Source: CAD feature listing. Evaluate the final solid. Frame: model axes, mm. Round coordinates to 2 decimals unless told otherwise and drop trailing zeros. Loops run counter-clockwise (first coordinate to the right, second up) from the corner with the lowest first, then second, coordinate; pieces in that order, holes last.
(1) Section D-D, the plane z = -207. Return the cut outline in (x, y).
(2) Section B-B, the plane z = -47. Return the cut outline in (x, y), plus the area to 3 significant figures.
(3) First-contact query: pin 1 Ø2.5 at (y, z) = (3, -191) entering from +X; pin 2 Ø2 at (x, y) = (28.5, 3) entering from -Z; pin 3 Ø1.4 at (y, z) = (1.5, -241.5) entering from -X. Flat tips, straight axial feed; report the tip coordinate or a pass-through.
(4) Section C-C, the plane x = 186. Return the cut outline in (y, z), plus the area to 3 significant figures.
(5) Section A-A, the plane x = 238. Return the cut outline in (y, z), plus the area to 3 significant figures.
(6) Material intervals for probe 1 along Z at (x, y) = (169, 1.35); probe 2 along Z at (x, y) = (97.5, 1.2); probe 3 along X at (y, z) = (3.6, -237.5), sorted ascending.
```python
from build123d import *

# Parameters (mm, degrees)
SKETCH1_W            = 254
SKETCH1_H            = 254
BOSS_EXTRUDE1_DEPTH  = 4.800000052
CUT_EXTRUDE2_DEPTH   = 360.242313767
CUT_EXTRUDE3_DEPTH   = 4.826
CUT_EXTRUDE5_DEPTH   = 4.826
CUT_EXTRUDE6_DEPTH   = 4.826
SKETCH16_OUTSIDE_W   = 327.848
SKETCH16_OUTSIDE_H   = 327.848
CUT_EXTRUDE8_DEPTH   = 360.242313767
SKETCH17_OUTSIDE_W   = 327.848
SKETCH17_OUTSIDE_H   = 327.848
CUT_EXTRUDE17_DEPTH  = 360.242313767
SKETCH18_OUTSIDE_W   = 327.848
SKETCH18_OUTSIDE_H   = 327.848
CUT_EXTRUDE18_DEPTH  = 216.155906991
SKETCH19_OUTSIDE_W   = 327.734
SKETCH19_OUTSIDE_H   = 327.834
SKETCH19_OUTSIDE_W_2 = 4.500000144
SKETCH19_OUTSIDE_H_2 = 16.933333333
CUT_EXTRUDE19_DEPTH  = 364.309275828
SKETCH32_W           = 4.800000052
SKETCH32_H           = 76.2
CUT_EXTRUDE22_DEPTH  = 25.4
CUT_EXTRUDE23_DEPTH  = 216.155906991
SKETCH34_W           = 4.800000052
SKETCH34_H           = 76.2
CUT_EXTRUDE24_DEPTH  = 25.4
SKETCH36_W           = 4.500000144
SKETCH36_H           = 16.933333333
CUT_EXTRUDE26_DEPTH  = 364.309275828
SKETCH37_W           = 4.500000144
SKETCH37_H           = 25.4
CUT_EXTRUDE27_DEPTH  = 360.171616324
SKETCH48_W           = 4.500000144
SKETCH48_H           = 25.4
CUT_EXTRUDE34_DEPTH  = 360.171616324
SKETCH50_R           = 1.4
CUT_EXTRUDE35_DEPTH  = 506.24041807
SKETCH51_R           = 1.1
CUT_EXTRUDE36_DEPTH  = 1021.904407936


with BuildPart() as part:
    # Sketch1 → Boss-Extrude1 (new body)
    with BuildSketch(Plane(origin=(0, 0, 0), x_dir=(1, 0, 0), z_dir=(0, 1, 0))):
        with Locations((127, 127)):
            Rectangle(SKETCH1_W, SKETCH1_H)
    extrude(amount=BOSS_EXTRUDE1_DEPTH)

    # Sketch4 → Cut-Extrude2 (cut, through all)
    with BuildSketch(Plane(origin=(0, 4.800000052, 0), x_dir=(1, 0, 0), z_dir=(0, 1, 0))):
        Polygon((76.2, 254), (0, 177.8), (0, 254), align=None)
    extrude(amount=-CUT_EXTRUDE2_DEPTH, mode=Mode.SUBTRACT)

    # Sketch5 → Cut-Extrude3 (cut)
    with BuildSketch(Plane(origin=(0, 4.800000052, 0), x_dir=(1, 0, 0), z_dir=(0, 1, 0))):
        Polygon((177.8, 254), (254, 177.8), (254, 254), align=None)
    extrude(amount=-CUT_EXTRUDE3_DEPTH, mode=Mode.SUBTRACT)

    # Sketch9 → Cut-Extrude5 (cut)
    with BuildSketch(Plane(origin=(0, 4.800000052, 0), x_dir=(1, 0, 0), z_dir=(0, 1, 0))):
        Polygon((0, 76.2), (0, 0), (76.2, 0), align=None)
    extrude(amount=-CUT_EXTRUDE5_DEPTH, mode=Mode.SUBTRACT)

    # Sketch11 → Cut-Extrude6 (cut)
    with BuildSketch(Plane(origin=(0, 4.800000052, 0), x_dir=(1, 0, 0), z_dir=(0, 1, 0))):
        Polygon((254, 76.2), (254, 0), (177.8, 0), align=None)
    extrude(amount=-CUT_EXTRUDE6_DEPTH, mode=Mode.SUBTRACT)

    # Sketch16 outside → Cut-Extrude8 (cut, through all)
    # profile 1 of 2: a face of its own
    with BuildSketch(Plane.XZ):
        with Locations((127, -127)):
            Rectangle(SKETCH16_OUTSIDE_W, SKETCH16_OUTSIDE_H)
        Polygon((254, -76.2), (177.8, 0), (76.2, 0), (0, -76.2), (0, -177.8), (76.2, -254), (177.8, -254), (254, -177.8), align=None, mode=Mode.SUBTRACT)
    # profile 2 of 2: a face of its own
    with BuildSketch(Plane.XZ):
        Polygon((154.05, -237.45), (152.4, -239.09956871), (152.4, -247.65), (157.899988492, -247.65), (157.899988492, -247.233680101), (157.899988492, -246.283680101), (157.899988492, -243.349999982), (157.899988492, -243.025), (157.899988492, -242.075), (157.899988492, -241.750000018), (157.899988492, -240.049999963), (157.899991793, -239.09957201), (156.249995092, -237.45), align=None)
    extrude(amount=-CUT_EXTRUDE8_DEPTH, mode=Mode.SUBTRACT)

    # Sketch17 outside → Cut-Extrude17 (cut, through all)
    # profile 1 of 2: a face of its own
    with BuildSketch(Plane.XZ):
        with Locations((127, -127)):
            Rectangle(SKETCH17_OUTSIDE_W, SKETCH17_OUTSIDE_H)
        Polygon((254, -76.2), (177.8, 0), (76.2, 0), (0, -76.2), (0, -177.8), (76.2, -254), (177.8, -254), (254, -177.8), align=None, mode=Mode.SUBTRACT)
    # profile 2 of 2: a face of its own
    with BuildSketch(Plane.XZ):
        Polygon((125.900002454, -218.4), (128.099997546, -218.4), (129.749994246, -220.04956871), (129.749994246, -220.999999963), (129.749994246, -222.700000018), (129.749994246, -223.025), (129.749994246, -223.975), (129.749994246, -224.299999982), (129.749994246, -227.233680101), (129.749994246, -228.183680101), (129.749994246, -228.6), (124.250005754, -228.6), (124.250005754, -228.183680101), (124.250005754, -228.15), (124.250005754, -227.233680101), (124.250005754, -224.299999982), (124.250005754, -223.975), (124.250005754, -223.025), (124.250005754, -222.700000018), (124.250005754, -220.999999963), (124.250005754, -220.04956871), align=None)
    extrude(amount=-CUT_EXTRUDE17_DEPTH, mode=Mode.SUBTRACT)

    # Sketch18 outside → Cut-Extrude18 (cut, through all)
    # profile 1 of 2: a face of its own
    with BuildSketch(Plane(origin=(166.661666982, 4.800000052, -135.988650526), x_dir=(1, 0, 0), z_dir=(0, 1, 0))):
        with Locations((-39.662, -8.989)):
            Rectangle(SKETCH18_OUTSIDE_W, SKETCH18_OUTSIDE_H)
        Polygon((-90.561667036, -135.988650526), (11.038332964, -135.988650526), (87.238332964, -59.788650526), (87.238332964, 41.811349474), (11.038332964, 118.011349474), (-90.561667036, 118.011349474), (-166.761667036, 41.811349474), (-166.761667036, -59.788650526), align=None, mode=Mode.SUBTRACT)
    # profile 2 of 2: a face of its own
    with BuildSketch(Plane(origin=(166.661666982, 4.800000052, -135.988650526), x_dir=(1, 0, 0), z_dir=(0, 1, 0))):
        Polygon((-65.461678544, 103.110918185), (-65.461678544, 111.661349474), (-70.961667036, 111.661349474), (-70.812431754, 103.061695826), (-69.211666982, 101.461349474), (-67.01167189, 101.461349474), align=None)
    extrude(amount=-CUT_EXTRUDE18_DEPTH, mode=Mode.SUBTRACT)

    # Sketch19 outside → Cut-Extrude19 (cut, through all)
    # profile 1 of 3: a face of its own
    with BuildSketch(Plane(origin=(277.632305151, 0, -234.288055689), x_dir=(1, 0, 0), z_dir=(0, -1, 0))):
        with Locations((-150.682, 107.288)):
            Rectangle(SKETCH19_OUTSIDE_W, SKETCH19_OUTSIDE_H)
        Polygon((-23.632305151, 158.088055689), (-99.832305151, 234.288055689), (-201.432305151, 234.288055689), (-277.632305151, 158.088055689), (-277.632305151, 56.488055689), (-201.432305151, -19.711944311), (-99.832305151, -19.711944311), (-23.632305151, 56.488055689), align=None, mode=Mode.SUBTRACT)
    # profile 2 of 3: a face of its own
    with BuildSketch(Plane(origin=(277.632305151, 0, -234.288055689), x_dir=(1, 0, 0), z_dir=(0, -1, 0))):
        with Locations((-54.584305223, 132.68805569)):
            Rectangle(SKETCH19_OUTSIDE_W_2, SKETCH19_OUTSIDE_H_2)
    # profile 3 of 3: a face of its own
    with BuildSketch(Plane(origin=(277.632305151, 0, -234.288055689), x_dir=(1, 0, 0), z_dir=(0, -1, 0))):
        with Locations((-54.584305223, 98.821389023)):
            Rectangle(SKETCH19_OUTSIDE_W_2, SKETCH19_OUTSIDE_H_2)
    cut_extrude19 = extrude(amount=-CUT_EXTRUDE19_DEPTH, mode=Mode.SUBTRACT)

    # Mirror2: Cut-Extrude19 across plane
    add(cut_extrude19.mirror(Plane(origin=(126.949999973, 0, 0), x_dir=(0, 0, 1), z_dir=(1, 0, 0))), mode=Mode.SUBTRACT)

    # Sketch32 → Cut-Extrude22 (cut)
    with BuildSketch(Plane(origin=(254, 6.738807757, -234.288055689), x_dir=(0, 1, 0), z_dir=(1, 0, 0))):
        with Locations((-4.338807731, 107.288055689)):
            Rectangle(SKETCH32_W, SKETCH32_H)
    extrude(amount=-CUT_EXTRUDE22_DEPTH, mode=Mode.SUBTRACT)

    # Sketch33 → Cut-Extrude23 (cut, through all)
    with BuildSketch(Plane(origin=(166.661666982, 0, -135.988650526), x_dir=(1, 0, 0), z_dir=(0, -1, 0))):
        Polygon((-42.582666982, 122.75320968), (-42.582666982, 125.686889799), (-42.582666982, 126.011889781), (-42.582666982, 126.961889781), (-42.582666982, 127.286889763), (-42.582666982, 128.986889819), (-42.582666982, 129.937321071), (-40.932670282, 131.586889781), (-38.73267519, 131.586889781), (-37.08267849, 129.937321071), (-37.08267849, 122.75320968), (-37.08267849, 121.80320968), (-37.08267849, 121.386889781), (-42.582666982, 121.386889781), (-42.582666982, 121.836889781), align=None)
    extrude(amount=-CUT_EXTRUDE23_DEPTH, mode=Mode.SUBTRACT)

    # Sketch34 → Cut-Extrude24 (cut)
    with BuildSketch(Plane(origin=(0, 6.738807757, -234.288055689), x_dir=(0, -1, 0), z_dir=(-1, 0, 0))):
        with Locations((4.338807731, 107.288055689)):
            Rectangle(SKETCH34_W, SKETCH34_H)
    extrude(amount=-CUT_EXTRUDE24_DEPTH, mode=Mode.SUBTRACT)

    # Sketch36 → Cut-Extrude26 (cut, through all)
    with BuildSketch(Plane(origin=(277.632305151, 0, -234.288055689), x_dir=(1, 0, 0), z_dir=(0, -1, 0))):
        with Locations((-110.770919354, 132.68805569)):
            Rectangle(SKETCH36_W, SKETCH36_H)
        with Locations((-110.770883223, 98.821389023)):
            Rectangle(SKETCH36_W, SKETCH36_H)
    cut_extrude26 = extrude(amount=-CUT_EXTRUDE26_DEPTH, mode=Mode.SUBTRACT)

    # Mirror3: Cut-Extrude26 across plane
    add(cut_extrude26.mirror(Plane(origin=(126.949999973, 0, 0), x_dir=(0, 0, 1), z_dir=(1, 0, 0))), mode=Mode.SUBTRACT)

    # Sketch37 → Cut-Extrude27 (cut, through all)
    with BuildSketch(Plane(origin=(0, 4.800000052, 0), x_dir=(1, 0, 0), z_dir=(0, 1, 0))):
        with Locations((127, 186.266666667)):
            Rectangle(SKETCH37_W, SKETCH37_H)
    extrude(amount=-CUT_EXTRUDE27_DEPTH, mode=Mode.SUBTRACT)

    # Sketch48 → Cut-Extrude34 (cut, through all)
    with BuildSketch(Plane(origin=(0, 0, 0), x_dir=(-1, 0, 0), z_dir=(0, -1, 0))):
        with Locations((-126.899999946, 46.566666667)):
            Rectangle(SKETCH48_W, SKETCH48_H)
    extrude(amount=-CUT_EXTRUDE34_DEPTH, mode=Mode.SUBTRACT)

    # Sketch50 → Cut-Extrude35 (cut, through all)
    with BuildSketch(Plane(origin=(0, 4.800000052, -436.783275868), x_dir=(1, 0, 0), z_dir=(0, 1, 0))):
        with Locations(Location((143.575, -330.426609202, 0), (0, 0, 270))):
            Circle(SKETCH50_R)
        with Locations(Location((110.425, -330.426609202, 0), (0, 0, 270))):
            Circle(SKETCH50_R)
        with Locations(Location((143.575, -374.976609202, 0), (0, 0, 270))):
            Circle(SKETCH50_R)
        with Locations(Location((110.425, -374.976609202, 0), (0, 0, 270))):
            Circle(SKETCH50_R)
    extrude(amount=-CUT_EXTRUDE35_DEPTH, mode=Mode.SUBTRACT)

    # Sketch51 → Cut-Extrude36 (cut, through all)
    with BuildSketch(Plane(origin=(0, 4.800000052, -988.816241862), x_dir=(1, 0, 0), z_dir=(0, 1, 0))):
        with Locations(Location((145.841662515, -863.378312681, 0), (0, 0, 270))):
            Circle(SKETCH51_R)
        with Locations(Location((106.721662515, -863.378312681, 0), (0, 0, 270))):
            Circle(SKETCH51_R)
        with Locations(Location((145.841662515, -913.928312681, 0), (0, 0, 270))):
            Circle(SKETCH51_R)
        with Locations(Location((106.721662515, -913.928312681, 0), (0, 0, 270))):
            Circle(SKETCH51_R)
    extrude(amount=-CUT_EXTRUDE36_DEPTH, mode=Mode.SUBTRACT)


solid = part.part
```
Output values:
1. outline: (29.2, 0) - (224.7, 0) - (224.7, 4.8) - (29.2, 4.8) - close
2. outline: (29.2, 0) - (124.65, 0) - (124.65, 4.8) - (29.2, 4.8) - close; (129.15, 0) - (224.7, 0) - (224.7, 4.8) - (129.15, 4.8) - close
2. area: 917 mm2
3. pin 1: stops at x = 241.95
3. pin 2: stops at z = -207.3
3. pin 3: stops at x = 63
4. outline: (0, -245.7) - (4.8, -245.7) - (4.8, -8.3) - (0, -8.3) - close
4. area: 1,140 mm2
5. outline: (0, -193.7) - (4.8, -193.7) - (4.8, -165.1) - (0, -165.1) - close; (0, -88.9) - (4.8, -88.9) - (4.8, -60.3) - (0, -60.3) - close
5. area: 275 mm2
6. probe 1: z = -254 to -143.93, -127 to -110.07, -93.13 to 0
6. probe 2: z = -254 to -247.65, -237.45 to 0
6. probe 3: x = 59.7 to 97.4, 99.7 to 154, 156.3 to 194.2
